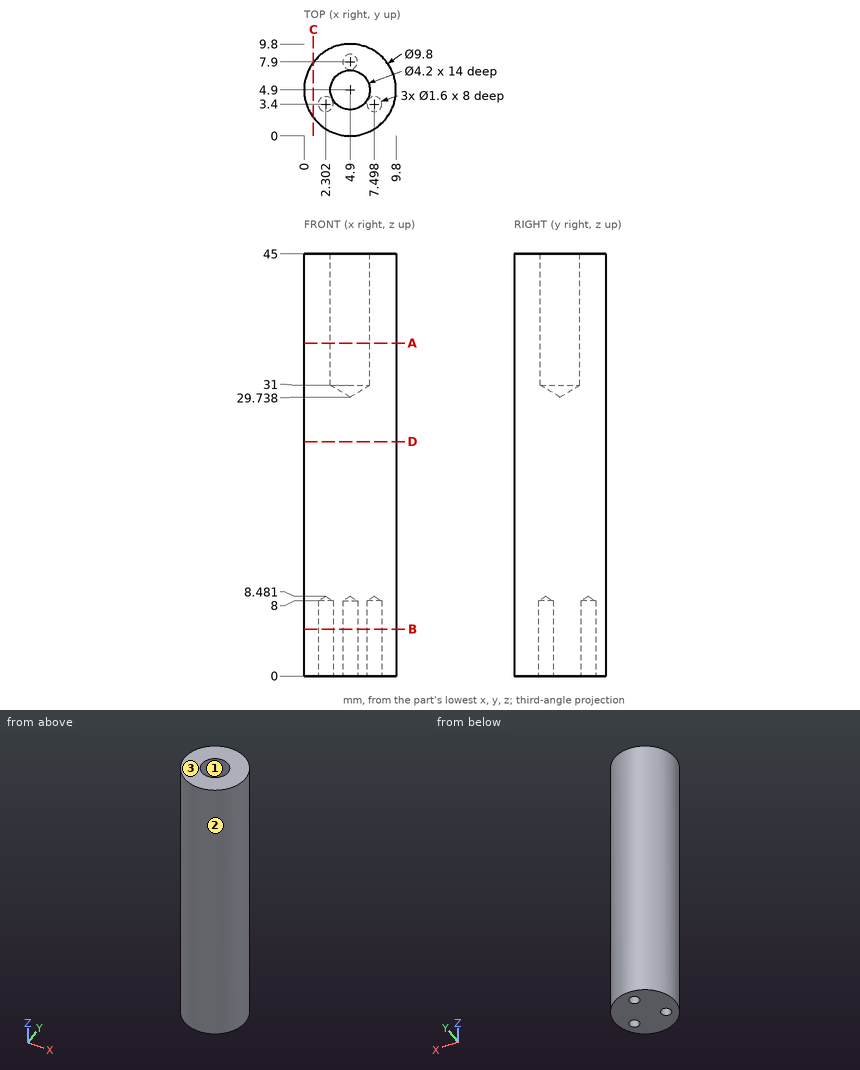
The figure shows three views and two pictorial views of one solid part (mm, origin at its lowest corner). Answer the questions. Give positions to 0.01 mm unless a question says otherwise; leave off trailing zeros. Write each loop counter-clockwise with the first axis right and the second up, starting at its lowest first coordinate (ties: lowest second). Pieces come first, ordered by that corner, then holes. Notation, with made-up numbers: (-18, 36) - (24, 36) arc R14 ccw to (24, 49) - close; hole circle Ø7 at (84.25, 31). An arc over 180 degrees is marked (long way). Use one line per item in the form item = value.
1. A cutting plane is placed at D-D (z = 25). Write down the section's boundary in (x, y), and give its area (3 significant figures).
Filled in:
outline = circle Ø9.8 at (4.9, 4.9)
area = 75.4 mm^2
2. A cutting plane is placed at B-B (z = 5). Write down the section's boundary in (x, y).
Filled in:
outline = circle Ø9.8 at (4.9, 4.9); hole circle Ø1.6 at (2.3, 3.4); hole circle Ø1.6 at (4.9, 7.9); hole circle Ø1.6 at (7.5, 3.4)
3. A cutting plane is placed at A-A (z = 35.5). Write down the section's boundary in (x, y).
Filled in:
outline = circle Ø9.8 at (4.9, 4.9); hole circle Ø4.2 at (4.9, 4.9)
4. This flat-tipped pin is pushed along its axis until it touches: pin 1 Ø3 at (y, z) = (2.5, 21.5) entering from +X. Where does it stop, or does it pass through?
Filled in:
pin_1 = 9.72
5. Determine the mould class of the marked faces 1, 2 and 3 for opening direction Y: released by +Y, released by -Y, zero draft, split by the parting line, or undercut.
Filled in:
face_1 = undercut
face_2 = split by the parting line
face_3 = zero draft
6. A cutting plane is placed at C-C (x = 1). Write down the section's boundary in (y, z), and give its area (3 significant figures).
Filled in:
outline = (1.93, 0) - (7.87, 0) - (7.87, 45) - (1.93, 45) - close
area = 267 mm^2
7. Consider L1, parallel to Y at x = 4.9, z = 5.75; L2, parallel to X at y = 3.4, z = 4.5 (1 decimal); L3, parallel to X at y = 7.9, z = 3.25 (1 decimal). Determine where each line is inside the solid, lowest interval first.
Filled in:
L1 = 0 to 7.1, 8.7 to 9.8
L2 = 0.2 to 1.5, 3.1 to 6.7, 8.3 to 9.6
L3 = 1 to 4.1, 5.7 to 8.8
